from build123d import *

# Parameters (mm, degrees)
SKETCH1_R           = 110
BOSS_EXTRUDE1_DEPTH = 3.5
SKETCH2_R           = 80
BOSS_EXTRUDE2_DEPTH = 0.001
SKETCH3_R           = 29.15
CUT_EXTRUDE1_DEPTH  = 4.5
SKETCH6_R           = 8.55
SKETCH6_R_2         = 5.3
CUT_EXTRUDE3_DEPTH  = 1.62
SKETCH7_R           = 5.3
CUT_EXTRUDE4_DEPTH  = 4.5
SKETCH8_R           = 80
CUT_EXTRUDE5_DEPTH  = 0.001


with BuildPart() as part:
    # Sketch1 → Boss-Extrude1 (new body)
    with BuildSketch(Plane.XY):
        Circle(SKETCH1_R)
    extrude(amount=BOSS_EXTRUDE1_DEPTH)

    # Sketch2 → Boss-Extrude2 (add)
    with BuildSketch(Plane(origin=(0, 0, 0), x_dir=(-1, 0, 0), z_dir=(0, 0, -1))):
        Circle(SKETCH2_R)
    extrude(amount=-BOSS_EXTRUDE2_DEPTH)

    # Sketch3 → Cut-Extrude1 (cut, through all)
    with BuildSketch(Plane(origin=(0, 0, 0), x_dir=(-1, 0, 0), z_dir=(0, 0, -1))):
        Circle(SKETCH3_R)
    extrude(amount=-CUT_EXTRUDE1_DEPTH, mode=Mode.SUBTRACT)

    # Sketch6 → Cut-Extrude3 (cut)
    with BuildSketch(Plane(origin=(0, 0, 0), x_dir=(-1, 0, 0), z_dir=(0, 0, -1))):
        with Locations((39.6625, 0)):
            Circle(SKETCH6_R)
        with Locations((39.6625, 0)):
            Circle(SKETCH6_R_2, mode=Mode.SUBTRACT)
        with Locations((-19.83125, -34.348732578)):
            Circle(SKETCH6_R)
        with Locations((-19.83125, -34.348732578)):
            Circle(SKETCH6_R_2, mode=Mode.SUBTRACT)
        with Locations((-19.83125, 34.348732578)):
            Circle(SKETCH6_R)
        with Locations((-19.83125, 34.348732578)):
            Circle(SKETCH6_R_2, mode=Mode.SUBTRACT)
    extrude(amount=-CUT_EXTRUDE3_DEPTH, mode=Mode.SUBTRACT)

    # Sketch7 → Cut-Extrude4 (cut, through all)
    with BuildSketch(Plane(origin=(0, 0, 0), x_dir=(-1, 0, 0), z_dir=(0, 0, -1))):
        with Locations((-19.83125, -34.348732578)):
            Circle(SKETCH7_R)
        with Locations((39.6625, 0)):
            Circle(SKETCH7_R)
        with Locations((-19.83125, 34.348732578)):
            Circle(SKETCH7_R)
    extrude(amount=-CUT_EXTRUDE4_DEPTH, mode=Mode.SUBTRACT)

    # Sketch8 → Cut-Extrude5 (cut)
    with BuildSketch(Plane(origin=(0, 0, 0), x_dir=(-1, 0, 0), z_dir=(0, 0, -1))):
        Circle(SKETCH8_R)
    extrude(amount=-CUT_EXTRUDE5_DEPTH, mode=Mode.SUBTRACT)


solid = part.part
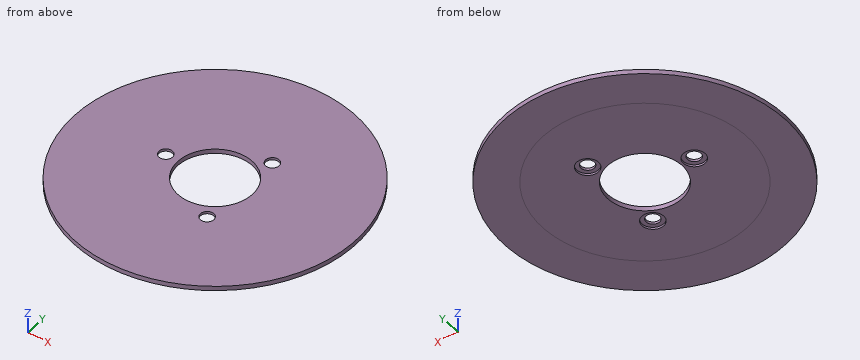
Work out the finished part from the listing and answer in its coordinate system (mm). Give positions to 0.01 mm unless a question says otherwise; leave off trailing zeros. Loops run counter-clockwise (first coordinate to the right, second up) from the corner with the lowest first, then second, coordinate; pieces in that order, holes last. Notation, with made-up numbers: M 58.5,-12 L 83.5,-12 A27 cw 83.5,10 Z; hole C 62,30.5 d9. An arc over 180 degrees is marked long. Use CSV: the item, a comma, the result in double quotes.
1) Find section C-C on z = 0.75. Write down the section's boundary in (x, y).
Answer:
outline,"C 0,0 d220; hole C -39.66,0 d17.1; hole C 0,0 d58.3; hole C 19.83,-34.35 d17.1; hole C 19.83,34.35 d17.1"
2) Consider L1, parallel to Y at x = -1.5, z = 2.3; L2, parallel to Y at x = 17, z = 1.55; L3, parallel to Z at x = 52.5, y = -11.5. Determine where each line is inside the solid, lowest interval first.
Answer:
L1,"-109.99 to -29.11, 29.11 to 109.99"
L2,"-108.68 to -42.42, -26.28 to -23.68, 23.68 to 26.28, 42.42 to 108.68"
L3,"0 to 3.5"
3) Given P1, Ø1, axis at y = -3, z = 2, coming from the -X side; P2, Ø17, axis at x = 19.83, y = 34.35, coming from the -Z side; P3, Ø10.5, axis at x = 19.83, y = -34.35, coming from the -Z side; P4, Ø19.5, axis at x = -39.66, y = 0, coming from the +Z side, each flat-ended and moving along its own axis, determine where each tip first touches the part or whether it passes through.
Answer:
P1,"x = -109.97"
P2,"z = 1.62"
P3,"through"
P4,"z = 3.5"
4) Find section B-B on y = 0. Give the number of separate pieces and of enclosed holes in the cut face, plus the area to 3 significant figures.
Answer:
separate pieces,"3"
enclosed holes,"0"
area,"518 mm^2"
